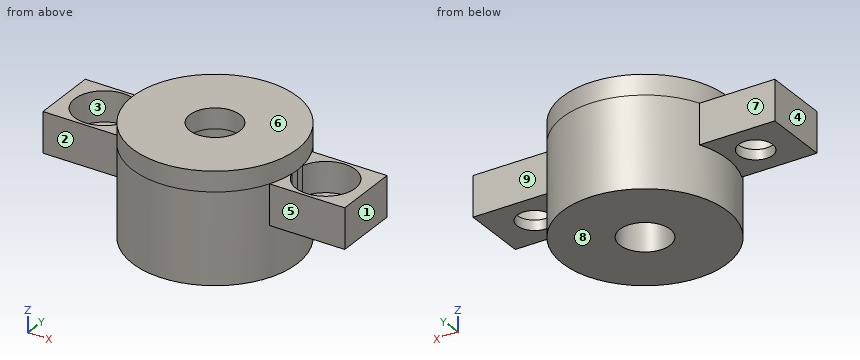
from build123d import *

# Parameters (mm, degrees)
CROQUIS1_R                   = 2.5
SALIENTE_EXTRUIR1_DEPTH      = 4
CROQUIS2_R                   = 1.7
CORTAR_EXTRUIR1_DEPTH        = 4
CROQUIS3_R                   = 2.95
CORTAR_EXTRUIR2_DEPTH        = 3
CROQUIS4_R                   = 8.2
CROQUIS4_R_2                 = 2.5
SALIENTE_EXTRUIR2_DEPTH      = 2
SALIENTE_EXTRUIR2_DEPTH_BACK = 9


with BuildPart() as part:
    # Croquis1 → Saliente-Extruir1 (new body)
    with BuildSketch(Plane.XY):
        with BuildLine():
            Line((-7.200520814, 3.25), (-15, 3.25))
            Line((-15, 3.25), (-15, -3.25))
            Line((-15, -3.25), (-7.200520814, -3.25))
            ThreePointArc((-7.200520814, -3.25), (0, -7.9), (7.200520814, -3.25))
            Line((7.200520814, -3.25), (15, -3.25))
            Line((15, -3.25), (15, 3.25))
            Line((15, 3.25), (7.200520814, 3.25))
            ThreePointArc((7.200520814, 3.25), (0, 7.9), (-7.200520814, 3.25))
        make_face()
        Circle(CROQUIS1_R, mode=Mode.SUBTRACT)
    extrude(amount=SALIENTE_EXTRUIR1_DEPTH)

    # Croquis2 → Cortar-Extruir1 (cut)
    with BuildSketch(Plane.XY.offset(4)):
        with Locations((-11, 0)):
            Circle(CROQUIS2_R)
        with Locations((11, 0)):
            Circle(CROQUIS2_R)
    extrude(amount=-CORTAR_EXTRUIR1_DEPTH, mode=Mode.SUBTRACT)

    # Croquis3 → Cortar-Extruir2 (cut)
    with BuildSketch(Plane.XY.offset(4)):
        with Locations((-11, 0)):
            Circle(CROQUIS3_R)
        with Locations((11, 0)):
            Circle(CROQUIS3_R)
    extrude(amount=-CORTAR_EXTRUIR2_DEPTH, mode=Mode.SUBTRACT)

    # Croquis4 → Saliente-Extruir2 (add, two sides)
    with BuildSketch(Plane.XY.offset(4)) as saliente_extruir2_sk:
        Circle(CROQUIS4_R)
        Circle(CROQUIS4_R_2, mode=Mode.SUBTRACT)
    extrude(amount=SALIENTE_EXTRUIR2_DEPTH)
    extrude(saliente_extruir2_sk.sketch, amount=-SALIENTE_EXTRUIR2_DEPTH_BACK)


solid = part.part
Input: part model. Units: mm. Frame: model coordinates. Face numbers are marked on the shaded views. A direction names the side the tool comes from. Coordinates: 2 decimals unless noted, no trailing zeros. Order: outer loops, then holes, each group sorted by start corner. A loop starts at its lowest first (then second) coordinate and runs counter-clockwise, first axis right, second up.
1. Access query for the marked faces 5, 6, 7, 8 and 9. Directions: +Z, -Z, +X, -X, +Y, -Y. A direction counts if a zero-diameter tool reaches every point of the face in a straight line with its end or side. Return the directions, or none.
Checked values:
face 5: +Z, -Z, +X, -Y
face 6: +Z, +X, -X, +Y, -Y
face 7: +Z, -Z, -X, +Y
face 8: -Z, +X, -X, +Y, -Y
face 9: +Z, -Z, +X, +Y
2. Ray query, line 1 along Y through (x, z) = (11, 0.8); line 2 along Y through (x, z) = (-11, 2.1); line 3 along X through (y, z) = (2, 0.25). Return the intervals inside material, ascending.
Checked values:
line 1: y = -3.25 to -1.7, 1.7 to 3.25
line 2: y = -3.25 to -2.95, 2.95 to 3.25
line 3: x = -15 to -1.5, 1.5 to 15
3. Cut plane D-D, the plane x = 0. Return loops of the section in (y, z).
Checked values:
outline: (-8.2, -5) - (-2.5, -5) - (-2.5, 6) - (-8.2, 6) - close; (2.5, -5) - (8.2, -5) - (8.2, 6) - (2.5, 6) - close
4. Cut plane B-B, the plane z = 3.25. Return loops of the section in (x, y).
Checked values:
outline: (-15, -3.25) - (-7.53, -3.25) arc R8.2 ccw to (7.53, -3.25) - (15, -3.25) - (15, 3.25) - (7.53, 3.25) arc R8.2 ccw to (-7.53, 3.25) - (-15, 3.25) - close; hole (-8.16, -0.8) arc R8.2 cw to (-8.16, 0.8) arc R2.95 ccw (long way) to start; hole circle Ø5 at (0, 0); hole (8.16, -0.8) arc R2.95 ccw (long way) to (8.16, 0.8) arc R8.2 cw to start
5. Contact query for flat-ended pins moving along their axis: P1, Ø4.5, axis at x = 12.5, z = 2, coming from the +Y side; P2, Ø4, axis at x = -11, y = 0, coming from the -Z side; P3, Ø1.7, axis at x = -12, y = -1, coming from the +Z side; P4, Ø1, axis at x = -11.5, y = -5, coming from the -Z side. Output: stop coordinate, or through.
Checked values:
P1: stops at y = 3.25
P2: stops at z = 0
P3: stops at z = 1
P4: passes through
6. Cut plane A-A, the plane x = 11. Return loops of the section in (y, z).
Checked values:
outline: (-3.25, 0) - (-1.7, 0) - (-1.7, 1) - (-2.95, 1) - (-2.95, 4) - (-3.25, 4) - close; (1.7, 0) - (3.25, 0) - (3.25, 4) - (2.95, 4) - (2.95, 1) - (1.7, 1) - close
7. Draft query along X for the marked faces 1, 2, 3 and 4. Return one class per face: +X half, -X half, draft (parallel to the pull), parting line (faces both ways), or undercut.
Checked values:
face 1: +X half
face 2: draft
face 3: undercut
face 4: -X half
8. Cut plane C-C, the plane z = 4.75. Return loops of the section in (x, y), plus the area to 3 significant figures.
Checked values:
outline: circle Ø16.4 at (0, 0); hole circle Ø5 at (0, 0)
area: 192 mm2
